Build history of the part. All positions in model axes, mm. Round coordinates to 2 decimals unless told otherwise and drop trailing zeros. Loops run counter-clockwise (first coordinate to the right, second up) from the corner with the lowest first, then second, coordinate; pieces in that order, holes last.
Autodesk Inventor part; units mm, degrees
ref_plane "YZ Plane" through (0, 0, 0) normal (1, 0, 0) x (0, 1, 0)
ref_plane "XZ Plane" through (0, 0, 0) normal (0, 1, 0) x (-1, 0, 0)
ref_plane "XY Plane" through (0, 0, 0) normal (0, 0, 1) x (1, 0, 0)
sketch "maiin" plane through (0, 0, 0) normal (0, 0, 1) x (1, 0, 0)
  circle A0 centre (-6.5018, 3.4753) radius 2.1844
  line L0 (-6.8203, 13.6107) -> (11.7059, 28.671)
  circle A1 centre (-27.2482, -11.1789) radius 2.1844
  arc A2 (-33.4335, -9.7418) -> (-25.8521, -17.3735) centre (-27.2482, -11.1789) ccw
  line L1 (34.75, -1.6563) -> (34.75, 23.7437)
  line L2 (15.7114, 30.0937) -> (28.4, 30.0937)
  circle A3 centre (28.4114, 23.7437) radius 2.1844
  circle A4 centre (28.4, -1.6563) radius 2.1844
  circle A5 centre (15.7114, 23.7437) radius 2.1844
  circle A6 centre (15.7, -1.6563) radius 2.1844
  arc A7 (34.75, 23.7437) -> (28.4, 30.0937) centre (28.4, 23.7437) ccw
  arc A8 (15.7114, 30.0937) -> (11.7059, 28.671) centre (15.7114, 23.7437) ccw
  arc A9 (28.4, -8.0063) -> (34.75, -1.6563) centre (28.4, -1.6563) ccw
  line L3 (28.4, -8.0063) -> (15.7114, -8.0063)
  line L4 (15.7114, -8.0063) -> (-25.8521, -17.3735)
  circle A10 centre (-24.886, 6.0028) radius 2.0955
  arc A11 (-24.886, 10.7653) -> (-29.5249, 7.0806) centre (-24.886, 6.0028) ccw
  line L5 (-33.4335, -9.7418) -> (-29.5249, 7.0806)
  line L6 (-14.8313, 10.7653) -> (-24.886, 10.7653)
  arc A12 (-14.8313, 10.7653) -> (-6.8203, 13.6107) centre (-14.8313, 23.4653) ccw
  point P0 (10.0881, 4.3711)
  point P1 (32.8902, 28.2338)
  dimension "d0" = 12.7
  dimension "d6" = 4.3688
  dimension "d9" = 12.7
  dimension "d10" = 25.4
  dimension "d11" = 12.7
  dimension "d12" = 25.4
  dimension "d14" = 4.191
  dimension "d15" = 9.525
  dimension "d16" = 12.7
sketch "Sketch1" plane through (0, 0, 0) normal (1, 0, 0) x (0, 1, 0)
  circle A0 centre (-34.9132, -20.2684) radius 2.1844
  line L0 (-35.2318, -10.133) -> (-16.7055, 4.9273)
  circle A1 centre (-55.6596, -34.9226) radius 2.1844
  arc A2 (-61.8449, -33.4855) -> (-54.2635, -41.1172) centre (-55.6596, -34.9226) ccw
  line L1 (6.3386, -25.4) -> (6.3386, 0)
  line L2 (-12.7, 6.35) -> (-0.0114, 6.35)
  circle A3 centre (0, 0) radius 2.1844
  circle A4 centre (-0.0114, -25.4) radius 2.1844
  circle A5 centre (-12.7, 0) radius 2.1844
  circle A6 centre (-12.7114, -25.4) radius 2.1844
  arc A7 (6.3386, 0) -> (-0.0114, 6.35) centre (-0.0114, 0) ccw
  arc A8 (-12.7, 6.35) -> (-16.7055, 4.9273) centre (-12.7, 0) ccw
  arc A9 (-0.0114, -31.75) -> (6.3386, -25.4) centre (-0.0114, -25.4) ccw
  line L3 (-0.0114, -31.75) -> (-12.7, -31.75)
  line L4 (-12.7, -31.75) -> (-54.2635, -41.1172)
  circle A10 centre (-53.2974, -17.7408) radius 2.0955
  arc A11 (-53.2974, -12.9783) -> (-57.9364, -16.663) centre (-53.2974, -17.7408) ccw
  line L5 (-61.8449, -33.4855) -> (-57.9364, -16.663)
  line L6 (-43.2428, -12.9783) -> (-53.2974, -12.9783)
  arc A12 (-43.2428, -12.9783) -> (-35.2318, -10.133) centre (-43.2428, -0.2783) ccw
extrude "Extrusion1" add sketch "Sketch1" along normal blind 1.5875
properties part number "Angle Brace Gusset" material "Acetal Resin, White"
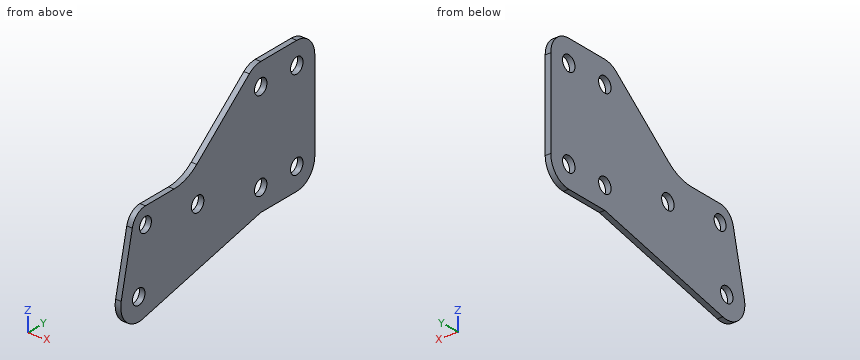
(1) Pin check, flat tips, straight feed: P1, Ø2.5, axis at y = -34.91, z = -20.27, coming from the +X side; P2, Ø0.8, axis at x = 1, y = -48.5, coming from the +Z side; P3, Ø0.8, axis at x = 0.5, y = -4, coming from the -Z side. Stop position of each tip, or through.
Responses:
P1: passes through
P2: stops at z = -12.98
P3: stops at z = -31.75
(2) Slice it at A-A on y = -52. List the corners of the cut face in (x, z), plus the area to 3 significant figures.
Responses:
outline: (0, -40.61) - (1.59, -40.61) - (1.59, -19.39) - (0, -19.39) - close; (0, -16.1) - (1.59, -16.1) - (1.59, -12.98) - (0, -12.98) - close
area: 38.6 mm2
(3) Slice it at B-B on x = 1. List the corners of the cut face in (y, z).
Responses:
outline: (-61.84, -33.49) arc R6.35 ccw to (-54.26, -41.12) - (-12.7, -31.75) - (-0.01, -31.75) arc R6.35 ccw to (6.34, -25.4) - (6.34, 0) arc R6.35 ccw to (-0.01, 6.35) - (-12.7, 6.35) arc R6.35 ccw to (-16.71, 4.93) - (-35.23, -10.13) arc R12.7 cw to (-43.24, -12.98) - (-53.3, -12.98) arc R4.76 ccw to (-57.94, -16.66) - close; hole circle Ø4.37 at (-55.66, -34.92); hole circle Ø4.19 at (-53.3, -17.74); hole circle Ø4.37 at (-34.91, -20.27); hole circle Ø4.37 at (-12.71, -25.4); hole circle Ø4.37 at (-12.7, 0); hole circle Ø4.37 at (-0.01, -25.4); hole circle Ø4.37 at (0, 0)
(4) Slice it at C-C on y = -8.5. List the corners of the cut face in (x, z), plus the area to 3 significant figures.
Responses:
outline: (0, -31.75) - (1.59, -31.75) - (1.59, 6.35) - (0, 6.35) - close
area: 60.5 mm2
(5) Probe line 1 (Z direction, x = 0.3, y = -12.7); line 2 (Y direction, x = 0.35, z = -1); line 3 (Z direction, x = 0.5, y = -12). List the from-to ranges inside material, lowest first.
Responses:
line 1: z = -31.75 to -27.58, -23.22 to -2.18, 2.18 to 6.35
line 2: y = -24 to -14.64, -10.76 to -1.94, 1.94 to 6.34
line 3: z = -31.75 to -27.47, -23.33 to -2.07, 2.07 to 6.35
(6) Slice it at D-D on z = -29. List the corners of the cut face in (x, y).
Responses:
outline: (0, -60.8) - (1.59, -60.8) - (1.59, 5.22) - (0, 5.22) - close
